Could you check a few things on this model? Use its own coordinates, in mm. Give positions to 0.01 mm unless a question says otherwise; leave off trailing zeros. Loops run counter-clockwise (first coordinate to the right, second up) from the corner with the lowest first, then second, coordinate; pieces in that order, holes last. Notation, with made-up numbers: M 77,27 L 102,27 A14 ccw 102,34 Z; hole C 25.25,30.25 d4. An arc over 180 degrees is marked long. Use CSV: the item, a comma, the result in double quotes.
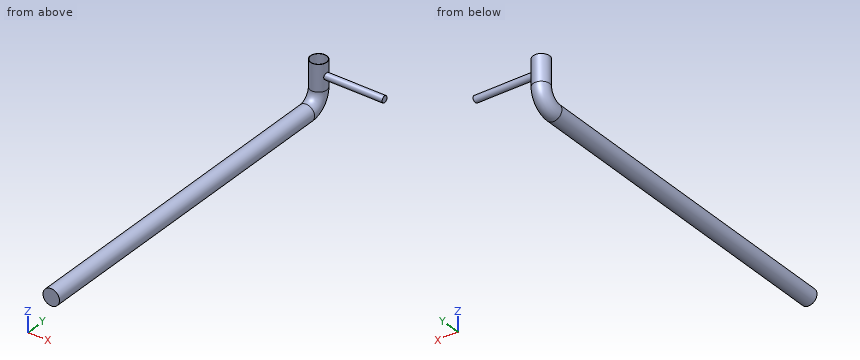
```python
from build123d import *

# Parameters (mm, degrees)
IZIM2_R                          = 2.5
BO_ALTMA3_T                      = -0.1
Y_KSEKLIK_EKSTR_ZYON2_REACH      = 88.496
Y_KSEKLIK_EKSTR_ZYON2_END_RADIUS = 2.5
IZIM4_R                          = 1


with BuildPart() as part:
    # Süpür1: sweep along a path in Çizim1
    with BuildLine(Plane(origin=(0, 0, 0), x_dir=(0, 0, -1), z_dir=(1, 0, 0))) as s_p_r1_path:
        Line((0, -28.77), (0, 75))
        ThreePointArc((0, 75), (-1.464466094, 78.535533906), (-5, 80))
        Line((-5, 80), (-13, 80))
    # Çizim2 → Süpür1 (sweep)
    with BuildSketch(Plane.XY.offset(13)):
        with Locations((0, 80)):
            Circle(IZIM2_R)
    sweep(path=s_p_r1_path.line)

    # İç Boşaltma3
    bo_altma3_openings = [part.faces().sort_by_distance(p)[0] for p in [
        (0, 80, 13),
    ]]
    offset(amount=BO_ALTMA3_T, openings=bo_altma3_openings, kind=Kind.INTERSECTION)

    # Yükseklik-Ekstrüzyon2: up to this cylinder (the profile starts outside it)
    y_kseklik_ekstr_zyon2_end = Plane(origin=(0, 80, 9), z_dir=(0, 0, 1)) * Cylinder(Y_KSEKLIK_EKSTR_ZYON2_END_RADIUS, 182.992, mode=Mode.PRIVATE)
    # Çizim4 → Yükseklik-Ekstrüzyon2 (add, up to the surface)
    with BuildSketch(Plane(origin=(20, 0, 0), x_dir=(0, 0, -1), z_dir=(1, 0, 0)), mode=Mode.PRIVATE) as y_kseklik_ekstr_zyon2_sk1:
        with Locations((-9, 80)):
            Circle(IZIM4_R)
    y_kseklik_ekstr_zyon2_tool1 = extrude(y_kseklik_ekstr_zyon2_sk1.sketch, amount=-Y_KSEKLIK_EKSTR_ZYON2_REACH, mode=Mode.PRIVATE) - y_kseklik_ekstr_zyon2_end
    add(y_kseklik_ekstr_zyon2_tool1.solids().sort_by_distance((20, 80, 9))[0])


solid = part.part
```
1. Please list where these lines run through material, in increasing order: line 1 (Z direction, x = 2, y = 53); line 2 (Y direction, x = 12, z = 8.75); line 3 (Y direction, x = 15.25, z = 8.25).
Outcome:
line 1,"-1.5 to -1.33, 1.33 to 1.5"
line 2,"79.03 to 80.97"
line 3,"79.34 to 80.66"
2. I want a section at A-A, the plane y = 65.5. List the corners of the cut face in (x, z) for me.
Outcome:
outline,"C 0,0 d5; hole C 0,0 d4.8"
3. I'm going to push flat-ended pins straight in: pin 1 Ø1 at (x, z) = (16, 11) entering from -Y; pin 2 Ø7.5 at (x, y) = (0, 80) entering from -Z; pin 3 Ø2 at (y, z) = (6, 1) entering from +X; pin 4 Ø5.5 at (x, z) = (-0.5, 1) entering from +Y. Where does each tip first touch, or does it pass through?
Outcome:
pin 1,"through"
pin 2,"z = -2.4"
pin 3,"x = 2.5"
pin 4,"y = 82.39"
4. I want a section at C-C, the plane z = 9. List the corners of the cut face in (x, y) for me.
Outcome:
outline,"M 2.29,79 L 20,79 L 20,81 L 2.29,81 A2.5 ccw long Z; hole C 0,80 d4.8"
5. I want a section at D-D, the plane x = 4.25. List the corners of the cut face in (y, z) for me, then the cut area to 3 significant figures.
Outcome:
outline,"C 80,9 d2"
area,"3.14 mm2"
6. I want a section at B-B, the plane x = 0. List the corners of the cut face in (y, z) for me, then the cut area to 3 significant figures.
Outcome:
outline,"M -28.77,-2.5 L 75,-2.5 A7.5 ccw 82.5,5 L 82.5,13 L 82.4,13 L 82.4,5 A7.4 cw 75,-2.4 L -28.67,-2.4 L -28.67,2.4 L 75,2.4 A2.6 ccw 77.6,5 L 77.6,13 L 77.5,13 L 77.5,5 A2.5 cw 75,2.5 L -28.77,2.5 Z"
area,"24.4 mm2"
